Answer from the drawing. Dimensions are ordinates in mm from the lowest x, y and z of the part. A direction names the side the tool comes from. Give positions to 0.01 mm unless a question says otherwise; leave off trailing zeros. Loops run counter-clockwise (first coordinate to the right, second up) from the corner with the lowest first, then second, coordinate; pieces in that order, holes last. Notation, with made-up numbers: (79.5, 9.5) - (116.5, 9.5) arc R26 cw to (116.5, 27.5) - close; hole circle Ø1 at (69, 57.25). An arc over 180 degrees is marked (long way). Put each result on its own line as item: value. Start each with the question number.
1. For the marked faces 1, 2, 3, 4 and 5, determine the directions among +Z, -Z, +X, -X, +Y, -Y from which every point of the face is accessible in a straight line to the end or side of a thin tool.
2. A cutting plane is placed at C-C, the plane z = 30. Determine the outline of the cut face in (x, y).
3. Given pin 1 Ø8 at (x, y) = (14.5, 53.5) entering from +Z; pin 2 Ø5 at (x, z) = (29, 13) entering from -Y; pin 3 Ø3 at (x, z) = (22.5, 32.5) entering from +Y; pin 4 Ø11 at (y, z) = (8.5, 33) entering from +X, each flat-ended and moving along its own axis, determine where each tip first touches the part or whether it passes through.
4. Consider L1, parallel to Z at x = 44.5, y = 36.5; L2, parallel to Z at x = 29, y = 19.5; L3, parallel to X at y = 8, z = 4. Determine where each line is inside the solid, lowest interval first. Write a range as from..to.
5. A cutting plane is placed at D-D, the plane y = 11.5. Determine the outline of the cut face in (x, z).
6. A cutting plane is placed at B-B, the plane x = 22.5. Determine the outline of the cut face in (y, z).
7. A cutting plane is placed at A-A, the plane y = 31.5. Determine the outline of the cut face in (x, z).
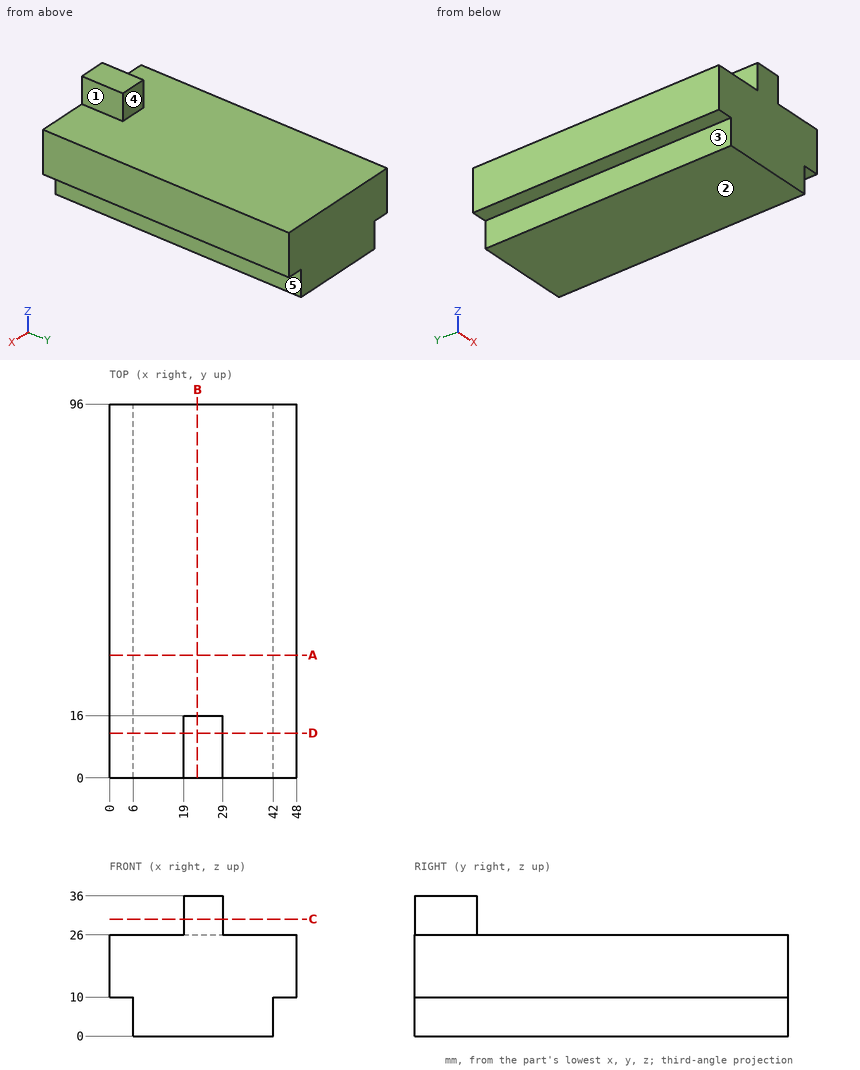
Return value:
1. face 1: +Z, +X, +Y, -Y
1. face 2: -Z, +X, -X, +Y, -Y
1. face 3: -Z, -X, +Y, -Y
1. face 4: +Z, +X, -X, +Y
1. face 5: -Z, +X, +Y, -Y
2. outline: (19, 0) - (29, 0) - (29, 16) - (19, 16) - close
3. pin 1: stops at z = 26
3. pin 2: stops at y = 0
3. pin 3: stops at y = 16
3. pin 4: stops at x = 29
4. L1: z = 10..26
4. L2: z = 0..26
4. L3: x = 6..42
5. outline: (0, 10) - (6, 10) - (6, 0) - (42, 0) - (42, 10) - (48, 10) - (48, 26) - (29, 26) - (29, 36) - (19, 36) - (19, 26) - (0, 26) - close
6. outline: (0, 0) - (96, 0) - (96, 26) - (16, 26) - (16, 36) - (0, 36) - close
7. outline: (0, 10) - (6, 10) - (6, 0) - (42, 0) - (42, 10) - (48, 10) - (48, 26) - (0, 26) - close
